from build123d import *

# Parameters (mm, degrees)
SKETCH_1_W          = 14
SKETCH_1_H          = 9
EXTRUDE_1_DEPTH     = 14
FILLET_1_R          = 1
SKETCH_3_R          = 1.75
CUT_EXTRUDE_2_DEPTH = 7
CUT_EXTRUDE_3_REACH = 12.874
SKETCH_4_R          = 0.95


with BuildPart() as part:
    # 草图1 → 凸台-拉伸1 (new body)
    with BuildSketch(Plane(origin=(0, 0, 0), x_dir=(1, 0, 0), z_dir=(0, 1, 0))):
        Rectangle(SKETCH_1_W, SKETCH_1_H)
    extrude(amount=EXTRUDE_1_DEPTH)

    # 圆角1
    fillet_1_edges = [part.edges().sort_by_distance(p)[0] for p in [
        (7, 7, 4.5),
        (-7, 7, 4.5),
        (-7, 7, -4.5),
        (7, 7, -4.5),
    ]]
    fillet(fillet_1_edges, radius=FILLET_1_R)

    # 草图3 → 切除-拉伸2 (cut)
    with BuildSketch(Plane(origin=(0, 14, 0), x_dir=(1, 0, 0), z_dir=(0, 1, 0))):
        with Locations(Location((-2.5, 0, 0), (0, 0, 270))):
            Circle(SKETCH_3_R)
        with Locations(Location((2.5, 0, 0), (0, 0, 90))):
            Circle(SKETCH_3_R)
    extrude(amount=-CUT_EXTRUDE_2_DEPTH, mode=Mode.SUBTRACT)

    # 草图4 → 切除-拉伸3 (cut, up to next)
    with BuildSketch(Plane(origin=(0, 7, 0), x_dir=(1, 0, 0), z_dir=(0, 1, 0)), mode=Mode.PRIVATE) as cut_extrude_3_sk1:
        with Locations(Location((-2.5, 0, 0), (0, 0, 270))):
            Circle(SKETCH_4_R)
    cut_extrude_3_tool1 = extrude(cut_extrude_3_sk1.sketch, amount=-CUT_EXTRUDE_3_REACH, mode=Mode.PRIVATE) & part.part
    # 草图4 → 切除-拉伸3 (cut, up to next)
    with BuildSketch(Plane(origin=(0, 7, 0), x_dir=(1, 0, 0), z_dir=(0, 1, 0)), mode=Mode.PRIVATE) as cut_extrude_3_sk2:
        with Locations(Location((2.5, 0, 0), (0, 0, 270))):
            Circle(SKETCH_4_R)
    cut_extrude_3_tool2 = extrude(cut_extrude_3_sk2.sketch, amount=-CUT_EXTRUDE_3_REACH, mode=Mode.PRIVATE) & part.part
    add(cut_extrude_3_tool1.solids().sort_by_distance((-2.5, 7, 0))[0], mode=Mode.SUBTRACT)
    add(cut_extrude_3_tool2.solids().sort_by_distance((2.5, 7, 0))[0], mode=Mode.SUBTRACT)


solid = part.part
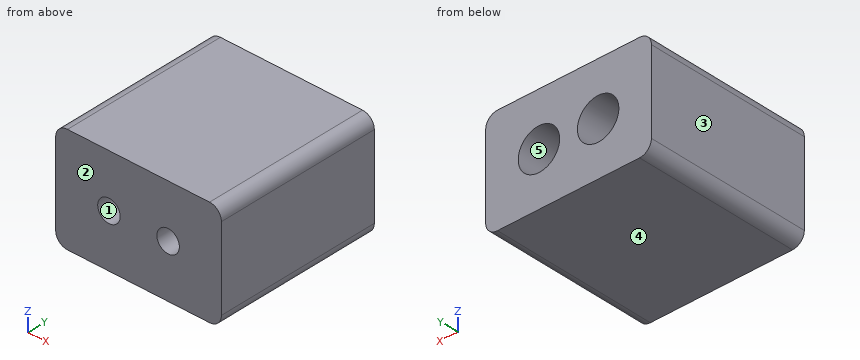
The model under review builds one solid part; all positions refer to its coordinate system, in mm. Face numbers are marked on the shaded views. A direction names the side the tool comes from. Coordinates: 2 decimals unless noted, no trailing zeros. Write each loop counter-clockwise with the first axis right and the second up, starting at its lowest first coordinate (ties: lowest second). Pieces come first, ordered by that corner, then holes. Notation, with made-up numbers: (53.25, -27) -> (62.25, -27) arc R9 cw to (62.25, -19) -> close; hole circle Ø4 at (-19, 76). An arc over 180 degrees is marked (long way). Answer in a Markdown table with one row per item.
1. Draft analysis for pull direction X (two halves, no side actions). For the marked faces 1, 2 and 3, state which applies: +X half, -X half, draft (parallel to the pull), parting line (faces both ways), or undercut.
Answers below:
| item | result |
|---|---|
| face 1 | undercut |
| face 2 | draft |
| face 3 | -X half |
2. Clearance check with flat-ended pins moving along their axes: pin 1 Ø1.1 at (x, z) = (-2.5, 0) entering from -Y; pin 2 Ø2 at (x, z) = (2.5, 0) entering from +Y. State where each tip first meets the part, or that it passes through.
Answers below:
| item | result |
|---|---|
| pin 1 | passes through |
| pin 2 | stops at y = 7 |
3. Wall thickness on probe 1 along X at (y, z) = (10.75, 0); probe 2 along X at (y, z) = (3.25, 0); probe 3 along Y at (x, z) = (3.75, -0.5): over which ranges is each line inside the solid? List them lowest first. Write a range as [from, to].
Answers below:
| item | result |
|---|---|
| probe 1 | x = [-7, -4.25], [-0.75, 0.75], [4.25, 7] |
| probe 2 | x = [-7, -3.45], [-1.55, 1.55], [3.45, 7] |
| probe 3 | y = [0, 7] |
4. We need section D-D, the plane y = 12.25. State the section outline as (x, z) points, and give its area (3 significant figures).
Answers below:
| item | result |
|---|---|
| outline | (-7, -3.5) arc R1 ccw to (-6, -4.5) -> (6, -4.5) arc R1 ccw to (7, -3.5) -> (7, 3.5) arc R1 ccw to (6, 4.5) -> (-6, 4.5) arc R1 ccw to (-7, 3.5) -> close; hole circle Ø3.5 at (-2.5, 0); hole circle Ø3.5 at (2.5, 0) |
| area | 106 mm^2 |
5. For the marked faces 4 and 5, list the 3-axis set-ups (+Z, -Z, +X, -X, +Y, -Y) from which the entire face can be reached by the end or side of a thin tool; tool diameter is ignored.
Answers below:
| item | result |
|---|---|
| face 4 | -Z, +X, -X, +Y, -Y |
| face 5 | +Y |
6. We need section A-A, the plane x = 2.5. State the section outline as (y, z) points, and give its area (3 significant figures).
Answers below:
| item | result |
|---|---|
| outline | (0, -4.5) -> (14, -4.5) -> (14, -1.75) -> (7, -1.75) -> (7, -0.95) -> (0, -0.95) -> close; (0, 0.95) -> (7, 0.95) -> (7, 1.75) -> (14, 1.75) -> (14, 4.5) -> (0, 4.5) -> close |
| area | 88.2 mm^2 |
7. We need section C-C, the plane y = 4. State the section outline as (x, z) points.
Answers below:
| item | result |
|---|---|
| outline | (-7, -3.5) arc R1 ccw to (-6, -4.5) -> (6, -4.5) arc R1 ccw to (7, -3.5) -> (7, 3.5) arc R1 ccw to (6, 4.5) -> (-6, 4.5) arc R1 ccw to (-7, 3.5) -> close; hole circle Ø1.9 at (-2.5, 0); hole circle Ø1.9 at (2.5, 0) |
8. We need section B-B, the plane z = 0. State the section outline as (x, y) points, and give its area (3 significant figures).
Answers below:
| item | result |
|---|---|
| outline | (-7, 0) -> (-3.45, 0) -> (-3.45, 7) -> (-4.25, 7) -> (-4.25, 14) -> (-7, 14) -> close; (-1.55, 0) -> (1.55, 0) -> (1.55, 7) -> (0.75, 7) -> (0.75, 14) -> (-0.75, 14) -> (-0.75, 7) -> (-1.55, 7) -> close; (3.45, 0) -> (7, 0) -> (7, 14) -> (4.25, 14) -> (4.25, 7) -> (3.45, 7) -> close |
| area | 120 mm^2 |
